from build123d import *

# Parameters (mm, degrees)
SKETCH1_R               = 12.1
BOSS_EXTRUDE1_DEPTH     = 3.5
SKETCH1_4_R             = 12.1
BOSS_EXTRUDE2_DEPTH     = 28.5
SKETCH3_W               = 4.5
SKETCH3_H               = 2.297717899
CUT_EXTRUDE1_DEPTH      = 1
CUT_EXTRUDE1_DEPTH_BACK = 29.5
SKETCH6_W               = 17
SKETCH6_H               = 5
BOSS_EXTRUDE4_DEPTH     = 15.48
SKETCH7_W               = 17
SKETCH7_H               = 3
BOSS_EXTRUDE5_DEPTH     = 21
SKETCH10_W              = 8
SKETCH10_H              = 15
CUT_EXTRUDE4_DEPTH      = 5
SKETCH12_W              = 17
SKETCH12_H              = 3
BOSS_EXTRUDE8_DEPTH     = 8
SKETCH9_R               = 1.5
CUT_EXTRUDE5_DEPTH      = 4
SKETCH13_W              = 10
SKETCH13_H              = 4
BOSS_EXTRUDE9_DEPTH     = 5
SKETCH15_W              = 5
SKETCH15_H              = 10
BOSS_EXTRUDE10_DEPTH    = 11.96
SKETCH17_W              = 5
SKETCH17_H              = 3
BOSS_EXTRUDE11_DEPTH    = 4
SKETCH16_W              = 5
SKETCH16_H              = 3
BOSS_EXTRUDE12_DEPTH    = 4
SKETCH20_W              = 10
SKETCH20_H              = 4
BOSS_EXTRUDE13_DEPTH    = 5
SKETCH22_W              = 5
SKETCH22_H              = 10
BOSS_EXTRUDE14_DEPTH    = 12.81
SKETCH26_W              = 5
SKETCH26_H              = 3
BOSS_EXTRUDE15_DEPTH    = 4
SKETCH25_W              = 5
SKETCH25_H              = 3
BOSS_EXTRUDE16_DEPTH    = 4
SKETCH27_R              = 1.5
CUT_EXTRUDE7_DEPTH      = 1.006326947
CUT_EXTRUDE7_DEPTH_BACK = 45.008836986
SKETCH28_R              = 1.5
CUT_EXTRUDE8_DEPTH      = 1
CUT_EXTRUDE8_DEPTH_BACK = 45.015163933


with BuildPart() as part:
    # Sketch1 → Boss-Extrude1 (new body)
    with BuildSketch(Plane.XY):
        Circle(SKETCH1_R)
    extrude(amount=BOSS_EXTRUDE1_DEPTH)

    # Sketch1<4> → Boss-Extrude2 (add)
    with BuildSketch(Plane.XY):
        with BuildLine():
            Line((10.134542374, 14.266781377), (-10.134542374, 14.266781377))
            ThreePointArc((-10.134542374, 14.266781377), (-12.405882938, 12.342773939), (-14.318281607, 10.061650551))
            Line((-14.318281607, 10.061650551), (-14.318281607, -10.061650551))
            ThreePointArc((-14.318281607, -10.061650551), (-12.406080895, -12.342574968), (-10.135, -14.266456287))
            Line((-10.135, -14.266456287), (10.135, -14.266456287))
            ThreePointArc((10.135, -14.266456287), (13.436306455, -11.212299891), (15.850202646, -7.417619301))
            Line((15.850202646, -7.417619301), (15.850202646, 7.417619301))
            ThreePointArc((15.850202646, 7.417619301), (13.436126626, 11.212515386), (10.134542374, 14.266781377))
        make_face()
        Circle(SKETCH1_4_R, mode=Mode.SUBTRACT)
    extrude(amount=BOSS_EXTRUDE2_DEPTH)

    # Sketch3 → Cut-Extrude1 (cut, two sides)
    with BuildSketch(Plane(origin=(0, 0, 0), x_dir=(-1, 0, 0), z_dir=(0, 0, -1))) as cut_extrude1_sk:
        with Locations((-0.45, 9.367922428)):
            Rectangle(SKETCH3_W, SKETCH3_H)
        with Locations((-0.45, -9.367922428)):
            Rectangle(SKETCH3_W, SKETCH3_H)
    extrude(amount=CUT_EXTRUDE1_DEPTH, mode=Mode.SUBTRACT)
    extrude(cut_extrude1_sk.sketch, amount=-CUT_EXTRUDE1_DEPTH_BACK, mode=Mode.SUBTRACT)

    # Sketch6 → Boss-Extrude4 (add)
    with BuildSketch(Plane(origin=(0, -14.266456287, 0), x_dir=(-1, 0, 0), z_dir=(0, -1, 0))):
        with Locations((0, -25)):
            Rectangle(SKETCH6_W, SKETCH6_H)
    extrude(amount=BOSS_EXTRUDE4_DEPTH)

    # Sketch7 → Boss-Extrude5 (add)
    with BuildSketch(Plane.XY.offset(27.5)):
        with Locations((0, -28.246456287)):
            Rectangle(SKETCH7_W, SKETCH7_H)
    extrude(amount=BOSS_EXTRUDE5_DEPTH)

    # Sketch10 → Cut-Extrude4 (cut, symmetric)
    with BuildSketch(Plane(origin=(0, -29.746456287, 0), x_dir=(-1, 0, 0), z_dir=(0, -1, 0))):
        with Locations((-0.050406815, -38.5)):
            Rectangle(SKETCH10_W, SKETCH10_H)
    extrude(amount=CUT_EXTRUDE4_DEPTH, both=True, mode=Mode.SUBTRACT)

    # Sketch12 → Boss-Extrude8 (add)
    with BuildSketch(Plane(origin=(0, -26.746456287, 0), x_dir=(1, 0, 0), z_dir=(0, 1, 0))):
        with Locations((0, -47)):
            Rectangle(SKETCH12_W, SKETCH12_H)
    extrude(amount=BOSS_EXTRUDE8_DEPTH)

    # Sketch9 → Cut-Extrude5 (cut, symmetric)
    with BuildSketch(Plane.XY.offset(48.5)):
        with Locations((-5.060010985, -23.75132246)):
            Circle(SKETCH9_R)
        with Locations((5.939989015, -23.75132246)):
            Circle(SKETCH9_R)
    extrude(amount=CUT_EXTRUDE5_DEPTH, both=True, mode=Mode.SUBTRACT)

    # Sketch13 → Boss-Extrude9 (add)
    with BuildSketch(Plane.ZY.offset(14.318281607)):
        with Locations((14, 0.308707646)):
            Rectangle(SKETCH13_W, SKETCH13_H)
    extrude(amount=BOSS_EXTRUDE9_DEPTH)

    # Sketch15 → Boss-Extrude10 (add)
    with BuildSketch(Plane(origin=(0, 2.308707646, 0), x_dir=(1, 0, 0), z_dir=(0, 1, 0))):
        with Locations((-16.818281607, -14)):
            Rectangle(SKETCH15_W, SKETCH15_H)
    extrude(amount=BOSS_EXTRUDE10_DEPTH)

    # Sketch17 → Boss-Extrude11 (add)
    with BuildSketch(Plane.XY.offset(19)):
        with Locations((-16.818281607, 12.768707646)):
            Rectangle(SKETCH17_W, SKETCH17_H)
    extrude(amount=BOSS_EXTRUDE11_DEPTH)

    # Sketch16 → Boss-Extrude12 (add)
    with BuildSketch(Plane(origin=(0, 0, 9), x_dir=(-1, 0, 0), z_dir=(0, 0, -1))):
        with Locations((16.818281607, 12.768707646)):
            Rectangle(SKETCH16_W, SKETCH16_H)
    extrude(amount=BOSS_EXTRUDE12_DEPTH)

    # Sketch20 → Boss-Extrude13 (add)
    with BuildSketch(Plane(origin=(15.850202646, 0, 0), x_dir=(0, 0, -1), z_dir=(1, 0, 0))):
        with Locations((-14, -0.547619301)):
            Rectangle(SKETCH20_W, SKETCH20_H)
    extrude(amount=BOSS_EXTRUDE13_DEPTH)

    # Sketch22 → Boss-Extrude14 (add)
    with BuildSketch(Plane(origin=(0, 1.452380699, 0), x_dir=(1, 0, 0), z_dir=(0, 1, 0))):
        with Locations((18.350202646, -14)):
            Rectangle(SKETCH22_W, SKETCH22_H)
    extrude(amount=BOSS_EXTRUDE14_DEPTH)

    # Sketch26 → Boss-Extrude15 (add)
    with BuildSketch(Plane.XY.offset(19)):
        with Locations((18.350202646, 12.762380699)):
            Rectangle(SKETCH26_W, SKETCH26_H)
    extrude(amount=BOSS_EXTRUDE15_DEPTH)

    # Sketch25 → Boss-Extrude16 (add)
    with BuildSketch(Plane(origin=(0, 0, 9), x_dir=(-1, 0, 0), z_dir=(0, 0, -1))):
        with Locations((-18.350202646, 12.762380699)):
            Rectangle(SKETCH25_W, SKETCH25_H)
    extrude(amount=BOSS_EXTRUDE16_DEPTH)

    # Sketch27 → Cut-Extrude7 (cut, two sides)
    with BuildSketch(Plane(origin=(0, 14.262380699, 0), x_dir=(1, 0, 0), z_dir=(0, 1, 0))) as cut_extrude7_sk:
        with Locations((18.350202646, -20.75)):
            Circle(SKETCH27_R)
        with Locations((18.350202646, -7.25)):
            Circle(SKETCH27_R)
    extrude(amount=CUT_EXTRUDE7_DEPTH, mode=Mode.SUBTRACT)
    extrude(cut_extrude7_sk.sketch, amount=-CUT_EXTRUDE7_DEPTH_BACK, mode=Mode.SUBTRACT)

    # Sketch28 → Cut-Extrude8 (cut, two sides)
    with BuildSketch(Plane(origin=(0, 14.268707646, 0), x_dir=(1, 0, 0), z_dir=(0, 1, 0))) as cut_extrude8_sk:
        with Locations((-16.818281607, -7.25)):
            Circle(SKETCH28_R)
        with Locations((-16.818281607, -20.75)):
            Circle(SKETCH28_R)
    extrude(amount=CUT_EXTRUDE8_DEPTH, mode=Mode.SUBTRACT)
    extrude(cut_extrude8_sk.sketch, amount=-CUT_EXTRUDE8_DEPTH_BACK, mode=Mode.SUBTRACT)


solid = part.part
Part model, mm, in its own coordinate system. A direction names the side the tool comes from. Coordinates: 2 decimals unless noted, no trailing zeros. Order: outer loops, then holes, each group sorted by start corner. A loop starts at its lowest first (then second) coordinate and runs counter-clockwise, first axis right, second up.
(1) Pull direction Y, two halves, no side cores. Call faces 5 (the face through (0, 14.267, 14)), 6 (the face through (2.7, -9, 2)), 7 (the face through (-17, 5, 9)): pulls with the +Y half, pulls with the -Y half, needs draft (parallel to the pull), parting line crosses it, or undercut.
Check sheet entries:
face 5: pulls with the +Y half
face 6: undercut
face 7: needs draft
(2) Probe L1, parallel to Z at x = 1.5, y = -24.5; L2, parallel to X at y = -0.5, z = 16.5; L3, parallel to Y at x = 0, z = 5. List the from-to ranges inside material, lowest first.
Check sheet entries:
L1: z = 22.5 to 27.5, 45.5 to 48.5
L2: x = -19.32 to -12.09, 12.09 to 20.85
L3: y = -14.27 to -12.1, 12.1 to 14.27
(3) Slice it at A-A, the plane z = 20.75. Write the cut outline in (x, y) (3 decimals).
Check sheet entries:
outline: (-19.318, 11.269) - (-18.318, 11.269) - (-18.318, 14.269) - (-19.318, 14.269) - close; (-15.318, 11.269) - (-14.318, 11.269) - (-14.318, 14.269) - (-15.318, 14.269) - close; (-14.318, -10.062) arc R17.5 ccw to (-10.135, -14.266) - (10.135, -14.266) arc R17.5 ccw to (15.85, -7.418) - (15.85, 7.418) arc R17.5 ccw to (10.135, 14.267) - (-10.135, 14.267) arc R17.5 ccw to (-14.318, 10.062) - close; (15.85, 11.262) - (16.85, 11.262) - (16.85, 14.262) - (15.85, 14.262) - close; (19.85, 11.262) - (20.85, 11.262) - (20.85, 14.262) - (19.85, 14.262) - close; hole circle Ø24.2 at (0, 0)
(4) Slice it at C-C, the plane z = 42.5. Write the cut outline in (x, y).
Check sheet entries:
outline: (-8.5, -29.75) - (-3.95, -29.75) - (-3.95, -26.75) - (-8.5, -26.75) - close; (4.05, -29.75) - (8.5, -29.75) - (8.5, -26.75) - (4.05, -26.75) - close
(5) Slice it at D-D, the plane y = 0. Write the cut outline in (x, z).
Check sheet entries:
outline: (-19.32, 9) - (-14.32, 9) - (-14.32, 0) - (15.85, 0) - (15.85, 9) - (20.85, 9) - (20.85, 19) - (15.85, 19) - (15.85, 28.5) - (12.1, 28.5) - (12.1, 3.5) - (-12.1, 3.5) - (-12.1, 28.5) - (-14.32, 28.5) - (-14.32, 19) - (-19.32, 19) - close
(6) Slice it at B-B, the plane x = 0. Write the cut outline in (y, z), and give its area (3 significant figures).
Check sheet entries:
outline: (-29.75, 22.5) - (-14.27, 22.5) - (-14.27, 0) - (-10.52, 0) - (-10.52, 3.5) - (-12.1, 3.5) - (-12.1, 28.5) - (-14.27, 28.5) - (-14.27, 27.5) - (-26.75, 27.5) - (-26.75, 31) - (-29.75, 31) - close; (-29.75, 46) - (-26.75, 46) - (-26.75, 45.5) - (-18.75, 45.5) - (-18.75, 48.5) - (-29.75, 48.5) - close; (-8.22, 0) - (8.22, 0) - (8.22, 3.5) - (-8.22, 3.5) - close; (10.52, 0) - (14.27, 0) - (14.27, 28.5) - (12.1, 28.5) - (12.1, 3.5) - (10.52, 3.5) - close
area: 312 mm2
(7) Pin check, flat tips, straight feed: pin 1 Ø4.5 at (x, z) = (18.5, 21) entering from -Y; pin 2 Ø1 at (y, z) = (-2, 7) entering from +X; pin 3 Ø8 at (y, z) = (-9.5, 28.5) entering from -X; pin 4 Ø2 at (x, y) = (5, -8.5) entering from -Z. Stop position of each tip, or through.
Check sheet entries:
pin 1: stops at y = -2.55
pin 2: stops at x = 15.85
pin 3: stops at x = -14.32
pin 4: stops at z = 0
(8) Tool access for faces 1 (the face through (0, -22, 22.5)), 2 (the face through (-1.8, 9, 2)), 3 (the face through (17.76, 11.262, 22.31)), 4 (the face through (11, 7, 28.5)): list every direction of +Z, -Z, +X, -X, +Y, -Y with a clear straight run to the whole face (end or side of a thin tool).
Check sheet entries:
face 1: -Z, +X, -X, -Y
face 2: +Z, -Z
face 3: +Z, +X, -Y
face 4: +Z, +X, -X, +Y
